Work out the finished part from the listing and answer in its coordinate system (mm). A direction names the side the tool comes from. Round coordinates to 2 decimals unless told otherwise and drop trailing zeros. Order: outer loops, then holes, each group sorted by start corner. A loop starts at its lowest first (then second) coordinate and runs counter-clockwise, first axis right, second up. Notation, with made-up numbers: (-34, 28) -> (0, 28) arc R21 cw to (0, 56) -> close; hole circle Ø1 at (67.25, -33.5). An arc over 180 degrees is marked (long way). Use one line per item in the form item = value.
Autodesk Inventor part; units mm, degrees
ref_plane "YZ Plane" through (0, 0, 0) normal (1, 0, 0) x (0, 1, 0)
ref_plane "XZ Plane" through (0, 0, 0) normal (0, 1, 0) x (-1, 0, 0)
ref_plane "XY Plane" through (0, 0, 0) normal (0, 0, 1) x (1, 0, 0)
sketch "Sketch1" plane through (0, 0, 0) normal (0, 0, 1) x (1, 0, 0)
  arc A0 (-1.6613, 2) -> (1.6613, 2) centre (0, 0) ccw
  line L0 (-1.6613, 2) -> (1.6613, 2)
  circle A1 centre (0, 0) radius 4.5
  dimension "d0" = 5.2
  dimension "d1" = 4.6
  dimension "d2" = 9
extrude "Extrusion1" add sketch "Sketch1" along normal blind 10
sketch "Sketch2" plane through (0, 0, 0) normal (0, 0, -1) x (-1, 0, 0)
  line L0 (1.7898, 3.1) -> (3.5796, 0)
  line L1 (3.5796, 0) -> (1.7898, -3.1)
  line L2 (1.7898, -3.1) -> (-1.7898, -3.1)
  line L3 (-1.7898, -3.1) -> (-3.5796, 0)
  line L4 (-3.5796, 0) -> (-1.7898, 3.1)
  line L5 (-1.7898, 3.1) -> (1.7898, 3.1)
  circle A0 centre (0, 0) radius 5
  dimension "d5" = 6.2
  dimension "d6" = 10
extrude "Extrusion2" add sketch "Sketch2" along normal blind 10
fillet "Fillet1" radius 2 2 edges at (-4.5, 0, 0) (5, 0, 0)
properties part number "Motor to hex coupler"
Item 1: Flat-ended cylindrical pins translate along their axes: P1, Ø2.5, axis at x = 0, z = 5.5, coming from the -Y side; P2, Ø3, axis at x = 1.5, y = 0, coming from the -Z side; P3, Ø5, axis at x = -3.5, z = -7, coming from the +Y side. Find the tip coordinate at first contact, or state that the pin passes through.
Findings:
P1 = -4.5
P2 = 0
P3 = 4.9
Item 2: Determine the mould class of faces 1 (the flat face through (0, 2, 5)), 2 (the cylindrical face through (1.08, 4.88, -5.24)), 3 (the flat face through (2, -2, 10)) for opening direction Y: released by +Y, released by -Y, zero draft, split by the parting line, or undercut.
Findings:
face_1 = undercut
face_2 = split by the parting line
face_3 = zero draft
Item 3: The part is cut by section C-C, the plane z = 2.5. Give the vertices of the cut face in (x, y), and give its area (3 significant figures).
Findings:
outline = circle Ø9 at (0, 0); hole (-1.66, 2) arc R2.6 ccw (long way) to (1.66, 2) -> close
area = 43.7 mm^2
Item 4: The part is cut by section A-A, the plane x = 0. Give the vertices of the cut face in (y, z).
Findings:
outline = (-5, -10) -> (-3.1, -10) -> (-3.1, 0) -> (-2.6, 0) -> (-2.6, 10) -> (-4.5, 10) -> (-4.5, 1.32) arc R2 cw to (-4.75, 0.35) arc R2 ccw to (-5, -0.61) -> close; (2, 0) -> (3.1, 0) -> (3.1, -10) -> (5, -10) -> (5, -0.61) arc R2 ccw to (4.75, 0.35) arc R2 cw to (4.5, 1.32) -> (4.5, 10) -> (2, 10) -> close
Item 5: Consider line 1 along Y through (x, z) = (0, -1); line 2 along Y through (x, z) = (-3.5, 0.5); line 3 along Y through (x, z) = (1, -1.5). Determine where each line is inside the solid, lowest interval first.
Findings:
line_1 = -5 to -3.1, 3.1 to 5
line_2 = -3.1 to 3.1
line_3 = -4.9 to -3.1, 3.1 to 4.9
Item 6: For faces 4 (the cylindrical face through (0.1, -2.6, 4.9)), 5 (the flat face through (2.672, -1.572, -4.93)), 6 (the cylindrical face through (-0.59, -4.46, 5.6)), determine the directions among +Z, -Z, +X, -X, +Y, -Y from which every point of the face is accessible in a straight line to the end or side of a thin tool.
Findings:
face_4 = +Z, -Z
face_5 = -Z
face_6 = +Z
Item 7: The part is cut by section B-B, the plane z = -5.5. Give the vertices of the cut face in (x, y).
Findings:
outline = circle Ø10 at (0, 0); hole (-3.58, 0) -> (-1.79, -3.1) -> (1.79, -3.1) -> (3.58, 0) -> (1.79, 3.1) -> (-1.79, 3.1) -> close
